Build history of the part. All positions in model axes, mm. Face numbers are marked on the shaded views. A direction names the side the tool comes from. Coordinates: 2 decimals unless noted, no trailing zeros. Write each loop counter-clockwise with the first axis right and the second up, starting at its lowest first coordinate (ties: lowest second). Pieces come first, ordered by that corner, then holes.
from build123d import *

# Parameters (mm, degrees)
F0_W     = 12
F0_H     = 18
F1_DEPTH = 1.8
F2_R     = 5.99999
F3_W     = 12
F3_H     = 5.5
F4_DEPTH = 0.6
F5_R     = 2.9
F6_DEPTH = 4.2
F7_R     = 1
F8_DEPTH = 25


# Not quite as in the source:
# - a fillet or chamfer is up to 0.001 mm smaller than in the source, because OpenCascade refuses the exact size


with BuildPart() as f1:
    # F0 (on Front) → F1 (new body)
    with BuildSketch(Plane.XZ):
        Rectangle(F0_W, F0_H)
    extrude(amount=F1_DEPTH)

    # F2 (radius 6 in the source; OpenCascade refuses exactly that, so slightly less here)
    f2_edges = [f1.edges().sort_by_distance(p)[0] for p in [
        (6, -0.9, -9),
        (-6, -0.9, -9),
    ]]
    fillet(f2_edges, radius=F2_R)

    # F3 (on face) → F4 (cut)
    with BuildSketch(Plane.XZ.offset(1.8)):
        with Locations((0, 6.25)):
            Rectangle(F3_W, F3_H)
    extrude(amount=-F4_DEPTH, mode=Mode.SUBTRACT)

    # F5 (on face) → F6 (join)
    with BuildSketch(Plane.XZ.offset(1.8)):
        with Locations((0, -3)):
            Circle(F5_R)
    extrude(amount=F6_DEPTH)

    # F7 (on face) → F8 (cut)
    with BuildSketch(Plane.XZ.offset(1.2)):
        with Locations((-3, 6.25)):
            Circle(F7_R)
        with Locations((3, 6.25)):
            Circle(F7_R)
    extrude(amount=-F8_DEPTH, mode=Mode.SUBTRACT)


solid = f1.part
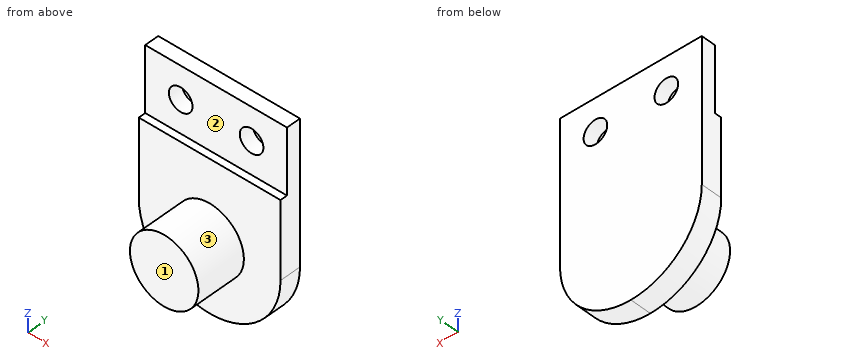
(1) Flat gauge pins, fed straight in: P1, Ø3, axis at x = 2, z = 6.5, coming from the -Y side; P2, Ø0.5, axis at x = 1, y = -1.5, coming from the +Z side. Where does each tip first touch, or does it go through?
(2) Slice it at D-D, the plane x = -3.75. List the corners of the cut face in (y, z).
(3) Slice it at C-C, the plane y = -5.45. List the corners of the cut face in (x, z).
(4) 3-axis set-ups, long thin cutter, end or side, ignore diameter. For the marked faces 1, 2 and 3: which of +Z, -Z, +X, -X, +Y, -Y reach the whole face in a straight line?
(5) Slice it at A-A, the plane z = 6.25. List the corners of the cut face in (x, y), and give its area (3 significant figures).
(6) Probe L1, parallel to Z at x = -3, y = -0.3; L2, parallel to Y at x = 2.75, z = 1.25; L3, parallel to Y at x = -3, z = 4.25. List the from-to ranges inside material, lowest first.
(7) Slice it at B-B, the plane x = 3.25. List the corners of the cut face in (y, z).
Results:
1. P1: stops at y = -1.2
1. P2: stops at z = 3.5
2. outline: (-1.8, -7.68) - (0, -7.68) - (0, 5.59) - (-1.2, 5.59) - (-1.2, 3.5) - (-1.8, 3.5) - close; (-1.2, 6.91) - (0, 6.91) - (0, 9) - (-1.2, 9) - close
3. outline: circle Ø5.8 at (0, -3)
4. face 1: +Z, -Z, +X, -X, -Y
4. face 2: +Z, +X, -X, -Y
4. face 3: -Y
5. outline: (-6, -1.2) - (-4, -1.2) - (-4, 0) - (-6, 0) - close; (-2, -1.2) - (2, -1.2) - (2, 0) - (-2, 0) - close; (4, -1.2) - (6, -1.2) - (6, 0) - (4, 0) - close
5. area: 9.60 mm2
6. L1: z = -8.2 to 5.25, 7.25 to 9
6. L2: y = -1.8 to 0
6. L3: y = -1.2 to 0
7. outline: (-1.8, -8.04) - (0, -8.04) - (0, 5.28) - (-1.2, 5.28) - (-1.2, 3.5) - (-1.8, 3.5) - close; (-1.2, 7.22) - (0, 7.22) - (0, 9) - (-1.2, 9) - close
